```python
from build123d import *

# Parameters (mm, degrees)
SKETCH16_R          = 10
BOSS_EXTRUDE4_DEPTH = 1.5
SKETCH17_R          = 5
BOSS_EXTRUDE5_DEPTH = 15
SKETCH18_R          = 2.5
CUT_EXTRUDE4_DEPTH  = 5
CUT_EXTRUDE7_DEPTH  = 3


with BuildPart() as part:
    # Sketch16 → Boss-Extrude4 (new body, symmetric)
    with BuildSketch(Plane.XY):
        Circle(SKETCH16_R)
    extrude(amount=BOSS_EXTRUDE4_DEPTH, both=True)

    # Sketch17 → Boss-Extrude5 (add)
    with BuildSketch(Plane.XY.offset(1.5)):
        Circle(SKETCH17_R)
    extrude(amount=BOSS_EXTRUDE5_DEPTH)

    # Sketch18 → Cut-Extrude4 (cut)
    with BuildSketch(Plane.XY.offset(16.5)):
        Circle(SKETCH18_R)
    extrude(amount=-CUT_EXTRUDE4_DEPTH, mode=Mode.SUBTRACT)

    # Sketch19 → Cut-Extrude7 (cut)
    with BuildSketch(Plane.XY.offset(16.5)):
        with BuildLine():
            ThreePointArc((-2.344526361, -0.867868735), (-2.165063509, 1.25), (-0.420666809, 2.464353756))
            Line((-0.420666809, 2.464353756), (-0.420666809, 4.982272517))
            ThreePointArc((-0.420666809, 4.982272517), (-4.330127019, 2.5), (-4.525107973, -2.126828116))
            Line((-4.525107973, -2.126828116), (-2.344526361, -0.867868735))
        make_face()
        with BuildLine():
            Line((0.420666809, 4.982272517), (0.420666809, 2.464353756))
            ThreePointArc((0.420666809, 2.464353756), (1.910715445, 1.612193068), (2.5, 0))
            ThreePointArc((2.5, 0), (2.460824649, -0.44084243), (2.344526361, -0.867868735))
            Line((2.344526361, -0.867868735), (4.525107973, -2.126828116))
            ThreePointArc((4.525107973, -2.126828116), (4.879832982, -1.089600875), (5, 0))
            ThreePointArc((5, 0), (3.681258891, 3.383538529), (0.420666809, 4.982272517))
        make_face()
        with BuildLine():
            Line((4.104441164, -2.855444402), (1.923859552, -1.596485021))
            ThreePointArc((1.923859552, -1.596485021), (0, -2.5), (-1.923859552, -1.596485021))
            Line((-1.923859552, -1.596485021), (-4.104441164, -2.855444402))
            ThreePointArc((-4.104441164, -2.855444402), (0, -5), (4.104441164, -2.855444402))
        make_face()
    extrude(amount=-CUT_EXTRUDE7_DEPTH, mode=Mode.SUBTRACT)


solid = part.part
```
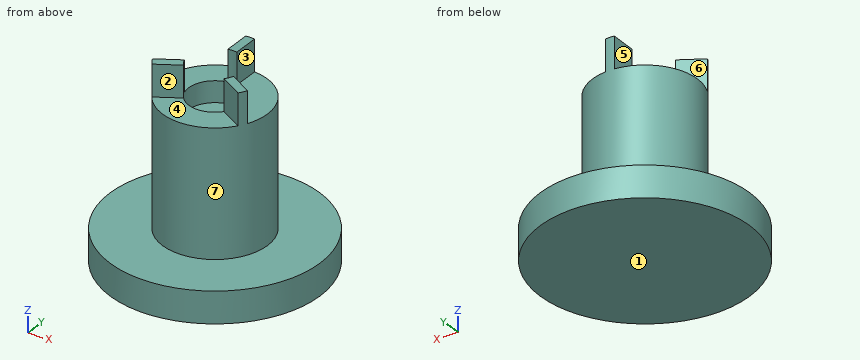
Check sheet for the modelled part. Datum: model origin and axes. Units: mm. Face numbers are marked on the shaded views. A direction names the side the tool comes from. Round coordinates to 2 decimals unless told otherwise and drop trailing zeros. Write each loop counter-clockwise with the first axis right and the second up, starting at its lowest first coordinate (ties: lowest second). Pieces come first, ordered by that corner, then holes. Notation, with made-up numbers: (8, -18.75) -> (47, -18.75) arc R16 cw to (47, 6.25) -> close; hole circle Ø7 at (-21.5, 39). An arc over 180 degrees is marked (long way). Put each result on its own line as item: value.
(1) Sectioned sample at D-D (z = 9.5). Enter the section's corners in (x, y).
Values found:
outline: circle Ø10 at (0, 0)
(2) Sectioned sample at A-A (z = 14.5). Enter the section's corners in (x, y), plus the area to 4 significant figures.
Values found:
outline: (-4.53, -2.13) arc R5 ccw to (-4.1, -2.86) -> (-1.92, -1.6) arc R2.5 cw to (-2.34, -0.87) -> close; (-0.42, 2.46) arc R2.5 cw to (0.42, 2.46) -> (0.42, 4.98) arc R5 ccw to (-0.42, 4.98) -> close; (1.92, -1.6) -> (4.1, -2.86) arc R5 ccw to (4.53, -2.13) -> (2.34, -0.87) arc R2.5 cw to start
area: 6.325 mm^2
(3) Sectioned sample at B-B (y = 0). Enter the section's corners in (x, z).
Values found:
outline: (-10, -1.5) -> (10, -1.5) -> (10, 1.5) -> (5, 1.5) -> (5, 13.5) -> (2.5, 13.5) -> (2.5, 11.5) -> (-2.5, 11.5) -> (-2.5, 13.5) -> (-5, 13.5) -> (-5, 1.5) -> (-10, 1.5) -> close
(4) Sectioned sample at C-C (x = 0). Enter the section's corners in (y, z), plus the area to 4 significant figures.
Values found:
outline: (-10, -1.5) -> (10, -1.5) -> (10, 1.5) -> (5, 1.5) -> (5, 16.5) -> (2.5, 16.5) -> (2.5, 11.5) -> (-2.5, 11.5) -> (-2.5, 13.5) -> (-5, 13.5) -> (-5, 1.5) -> (-10, 1.5) -> close
area: 177.5 mm^2
(5) Tool access check on the marked faces 4, 5, 6 and 7. Record the directions out of +Z, -Z, +X, -X, +Y, -Y that give a thin tool (end or side, any length) a straight path to the whole face; none if there is none.
Values found:
face 4: +Z, -Y
face 5: +Z, -X, +Y, -Y
face 6: +Z, -X, +Y
face 7: +Z
(6) Go/stop test with flat-tipped pins: pin 1 Ø6.5 at (x, y) = (0, 0) entering from +Z; pin 2 Ø1.7 at (x, y) = (0, -3) entering from +Z; pin 3 Ø0.8 at (y, z) = (4, 14.5) entering from +X; pin 4 Ø8 at (y, z) = (-4.5, 10.5) entering from -X. Record where each tip stops, or that it passes through.
Values found:
pin 1: stops at z = 16.5
pin 2: stops at z = 13.5
pin 3: stops at x = 0.42
pin 4: stops at x = -4.97
(7) Material ranges on line 1 (X direction, y = 0, z = 12.5); line 2 (Z direction, x = -2, y = 2); line 3 (Y direction, x = 1.5, z = 12), recorded low to high.
Values found:
line 1: x = -5 to -2.5, 2.5 to 5
line 2: z = -1.5 to 13.5
line 3: y = -4.77 to -2, 2 to 4.77
(8) Mould release check, pull along X, two halves, no side actions. Record for the marked faces 1, 2 and 3: released by +X, released by -X, zero draft, split by the parting line, or undercut.
Values found:
face 1: zero draft
face 2: undercut
face 3: released by +X
